Source: CAD feature listing. Evaluate the final solid. Frame: model axes, mm. Face numbers are marked on the shaded views. A direction names the side the tool comes from. Coordinates: 2 decimals unless noted, no trailing zeros. Loops run counter-clockwise (first coordinate to the right, second up) from the corner with the lowest first, then second, coordinate; pieces in that order, holes last.
Item 1: Section query C-C, the plane x = 10.75. Return the cut outline in (y, z).
Item 2: Reachability of the marked faces 1, 2 and 3 from +Z, -Z, +X, -X, +Y, -Y: full face, straight path, thin tool, end or side. Return the list, or none.
Item 3: Pull-direction query (Y, two-part tool) for the marked faces 4, 5 and 6; classes: +Y half, -Y half, draft (parallel to the pull), parting line (faces both ways), or undercut.
Item 4: Section query B-B, the plane y = 50.8. Return the cut outline in (x, z).
Item 5: Line query: probe 1 along Z at (x, y) = (5, 50.8); probe 2 along Y at (x, z) = (2.5, -38.1) (3 decimals); probe 3 along X at (y, z) = (19, -38). Output: solid intervals per line, ascending.
Item 6: Section query D-D, the plane y = 30.5. Return the cut outline in (x, z), then the cut area to 3 significant figures.
Item 7: Section query A-A, the plane z = -63.5. Return the cut outline in (x, y), then the cut area to 3 significant figures.
Item 8: Pin query (flat end, axial travel): pin 1 Ø4 at (x, z) = (4, -57.5) entering from -Y; pin 2 Ø6 at (x, y) = (5, -9) entering from +Z; pin 3 Ø10 at (y, z) = (50.8, -63.5) entering from -X; pin 4 Ø4 at (x, y) = (5.5, -12.5) entering from -Z. Return the tip coordinate at first contact, or that it passes through.
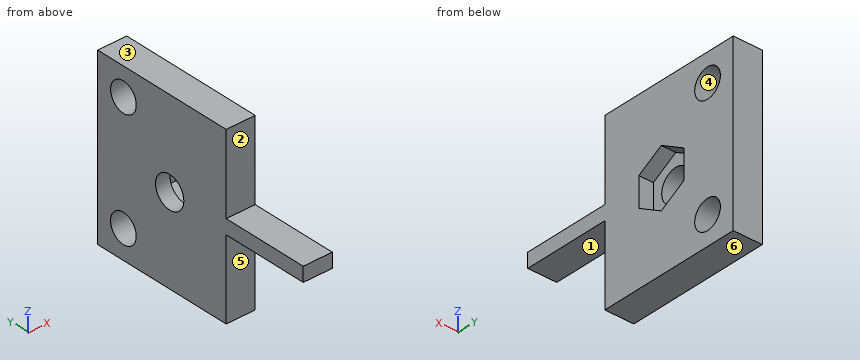
Autodesk Inventor part; units mm, degrees
ref_plane "YZ Plane" through (0, 0, 0) normal (1, 0, 0) x (0, 1, 0)
ref_plane "XZ Plane" through (0, 0, 0) normal (0, 1, 0) x (-1, 0, 0)
ref_plane "XY Plane" through (0, 0, 0) normal (0, 0, 1) x (1, 0, 0)
sketch "Sketch1" plane through (0, 0, 0) normal (1, 0, 0) x (0, 1, 0)
  circle A0 centre (27.94, -38.1) radius 6.985 construction
  circle A1 centre (50.8, -12.0577) radius 6.35
  line L0 (63.5, 0.1606) -> (50.8, 0.1606) construction
  line L1 (50.8, 0.1606) -> (50.8, -12.5394) construction
  line L2 (50.8, -12.5394) -> (63.5, -12.5394) construction
  line L3 (63.5, -12.5394) -> (63.5, 0.1606) construction
  circle A2 centre (50.8, -63.5) radius 6.35
  line L4 (16.8275, -31.6842) -> (27.94, -25.2684) construction
  line L5 (27.94, -25.2684) -> (39.0525, -31.6842) construction
  line L6 (39.0525, -31.6842) -> (39.0525, -44.5158) construction
  line L7 (39.0525, -44.5158) -> (27.94, -50.9316) construction
  line L8 (27.94, -50.9316) -> (16.8275, -44.5158) construction
  line L9 (16.8275, -44.5158) -> (16.8275, -31.6842) construction
  line L10 (0, -34.7644) -> (-38.1, -34.7644)
  line L11 (-38.1, -34.7644) -> (-38.1, -41.1144)
  line L12 (-38.1, -41.1144) -> (0, -41.1144)
  line L13 (63.5, 0.1606) -> (0, 0.1606)
  line L14 (0, -76.0394) -> (63.5, -76.0394)
  line L15 (63.5, -76.0394) -> (63.5, 0.1606)
  line L16 (0, 0.1606) -> (0, -34.7644)
  line L17 (0, -41.1144) -> (0, -76.0394)
  line L18 (0, -37.9394) -> (27.94, -37.9394) construction
  line L19 (0, -37.9394) -> (27.94, -37.9394) construction
  point P0 (0, 0)
  dimension "d9" = 13.97
  dimension "d12" = 12.7
  dimension "d13" = 12.7
  dimension "d18" = 22.225
  dimension "d21" = 38.1
  dimension "d22" = 6.35
  dimension "d23" = 63.5
  dimension "d24" = 76.2
  dimension "d38" = 38.1
  dimension "d41" = 27.94
  dimension "d42" = 0
  dimension "d43" = 34.925
  dimension "d44" = 38.1
extrude "Extrusion3" add sketch "Sketch1" along normal blind 12.7
sketch "Sketch2" plane through (12.7, 0, 0) normal (1, 0, 0) x (0, 0, -1)
  line L0 (0, 0) -> (38.1, 0) construction
  line L1 (38.1, 0) -> (38.1, 27.94) construction
  line L2 (31.6842, 16.8275) -> (25.2684, 27.94)
  line L3 (25.2684, 27.94) -> (31.6842, 39.0525)
  line L4 (31.6842, 39.0525) -> (44.5158, 39.0525)
  line L5 (44.5158, 39.0525) -> (50.9316, 27.94)
  line L6 (50.9316, 27.94) -> (44.5158, 16.8275)
  line L7 (44.5158, 16.8275) -> (31.6842, 16.8275)
  point P0 (38.1, 16.8275)
  dimension "d29" = 38.1
  dimension "d30" = 27.94
  dimension "d31" = 90
  dimension "d32" = 22.225
extrude "Extrusion4" cut sketch "Sketch2" against normal blind 6.35
sketch "Sketch3" plane through (6.35, 0, 0) normal (1, 0, 0) x (0, 0, -1)
  line L0 (25.2684, 27.94) -> (31.6842, 39.0525) construction
  line L1 (31.6842, 39.0525) -> (44.5158, 16.8275) construction
  circle A0 centre (38.1, 27.94) radius 6.985
  point P0 (0, 0)
  dimension "d35" = 13.97
extrude "Extrusion5" cut sketch "Sketch3" along normal through all both and the other way through all
equation "\"d38\" = d21"
properties part number "Holder" material "PVC-Piping"
Verdict:
1. outline: (-38.1, -41.11) - (0, -41.11) - (0, -76.04) - (63.5, -76.04) - (63.5, 0.16) - (0, 0.16) - (0, -34.76) - (-38.1, -34.76) - close; hole (16.83, -44.52) - (27.94, -50.93) - (39.05, -44.52) - (39.05, -31.68) - (27.94, -25.27) - (16.83, -31.68) - close; hole circle Ø12.7 at (50.8, -63.5); hole circle Ø12.7 at (50.8, -12.06)
2. face 1: -Z, +X, -X, -Y
2. face 2: +Z, +X, -X, -Y
2. face 3: +Z, +X, -X, +Y, -Y
3. face 4: undercut
3. face 5: -Y half
3. face 6: draft
4. outline: (0, -76.04) - (12.7, -76.04) - (12.7, -69.85) - (0, -69.85) - close; (0, -57.15) - (12.7, -57.15) - (12.7, -18.41) - (0, -18.41) - close; (0, -5.71) - (12.7, -5.71) - (12.7, 0.16) - (0, 0.16) - close
5. probe 1: z = -76.04 to -69.85, -57.15 to -18.41, -5.71 to 0.16
5. probe 2: y = -38.1 to 20.955, 34.925 to 63.5
5. probe 3: x = 0 to 6.35
6. outline: (0, -76.04) - (12.7, -76.04) - (12.7, -49.45) - (6.35, -49.45) - (6.35, -44.6) - (0, -44.6) - close; (0, -31.6) - (6.35, -31.6) - (6.35, -26.75) - (12.7, -26.75) - (12.7, 0.16) - (0, 0.16) - close
6. area: 741 mm2
7. outline: (0, 0) - (12.7, 0) - (12.7, 44.45) - (0, 44.45) - close; (0, 57.15) - (12.7, 57.15) - (12.7, 63.5) - (0, 63.5) - close
7. area: 645 mm2
8. pin 1: stops at y = 0
8. pin 2: stops at z = -34.76
8. pin 3: passes through
8. pin 4: stops at z = -41.11
